```python
from build123d import *

# Parameters (mm, degrees)
F0_W     = 482.6
F0_H     = 76.2
F1_DEPTH = 6.35
F2_W     = 25.4
F2_H     = 6.35
F3_DEPTH = 6.35
F4_W     = 6.35
F4_H     = 12.7
F5_DEPTH = 6.35


with BuildPart() as f1:
    # F0 (on Right) → F1 (new body)
    with BuildSketch(Plane.YZ):
        Rectangle(F0_W, F0_H)
    extrude(amount=F1_DEPTH)

    # F2 (on face) → F3 (cut, through all)
    with BuildSketch(Plane.YZ.offset(6.35)):
        with Locations((-228.6, -34.925)):
            Rectangle(F2_W, F2_H)
        with Locations((-177.8, -34.925)):
            Rectangle(F2_W, F2_H)
        with Locations((-127, -34.925)):
            Rectangle(F2_W, F2_H)
        with Locations((-76.2, -34.925)):
            Rectangle(F2_W, F2_H)
        with Locations((-25.4, -34.925)):
            Rectangle(F2_W, F2_H)
        with Locations((25.4, -34.925)):
            Rectangle(F2_W, F2_H)
        with Locations((76.2, -34.925)):
            Rectangle(F2_W, F2_H)
        with Locations((127, -34.925)):
            Rectangle(F2_W, F2_H)
        with Locations((177.8, -34.925)):
            Rectangle(F2_W, F2_H)
        with Locations((228.6, -34.925)):
            Rectangle(F2_W, F2_H)
    extrude(amount=-F3_DEPTH, mode=Mode.SUBTRACT)

    # F4 (on face) → F5 (cut, through all)
    with BuildSketch(Plane.YZ.offset(6.35)):
        with Locations((-238.125, 31.75)):
            Rectangle(F4_W, F4_H)
        with Locations((-238.125, 6.35)):
            Rectangle(F4_W, F4_H)
        with Locations((-238.125, -19.05)):
            Rectangle(F4_W, F4_H)
        with Locations((-28.575, 31.75)):
            Rectangle(F4_W, F4_H)
        with Locations((-28.575, 6.35)):
            Rectangle(F4_W, F4_H)
        with Locations((-28.575, -19.05)):
            Rectangle(F4_W, F4_H)
        with Locations((238.125, 31.75)):
            Rectangle(F4_W, F4_H)
        with Locations((238.125, 6.35)):
            Rectangle(F4_W, F4_H)
        with Locations((238.125, -19.05)):
            Rectangle(F4_W, F4_H)
    extrude(amount=-F5_DEPTH, mode=Mode.SUBTRACT)


solid = f1.part
```
Model file for the job. Use its own axes, mm. Give positions to 0.01 mm unless a question says otherwise; leave off trailing zeros. Write each loop counter-clockwise with the first axis right and the second up, starting at its lowest first coordinate (ties: lowest second). Pieces come first, ordered by that corner, then holes. Notation, with made-up numbers: (-26.75, -29.5) -> (-20.75, -29.5) arc R11 ccw to (-20.75, -14.5) -> close; hole circle Ø10 at (-0.5, -37). An arc over 180 degrees is marked (long way). Use CSV: the item, a comma, the result in double quotes. Start each with the question number.
1) Pin check, flat tips, straight feed: P1, Ø3, axis at x = 2.5, z = -22, coming from the -Y side; P2, Ø10, axis at y = 105, z = 12, coming from the -X side; P3, Ø1.9, axis at x = 2, y = -27, coming from the -Z side; P4, Ø1.9, axis at x = 4, y = -28.5, coming from the +Z side. Stop position of each tip, or through.
2) Drill centre lines: L1, parallel to Y at x = 1, z = 3; L2, parallel to Z at x = 3, y = 13.5. Where is each one in solid material? Low to high.
3) Cut at C-C on y = 29. List the corners of the cut face in (x, z), plus the area to 3 significant figures.
4) Cut at B-B on x = 5.25. Count the separate pieces of the cut face and the enclosed holes in it, plus the area to 3 significant figures.
5) Cut at A-A on z = -17.5. List the corners of the cut face in (x, y).
Final values:
1,P1,"stops at y = -234.95"
1,P2,"stops at x = 0"
1,P3,"stops at z = -31.75"
1,P4,"stops at z = 25.4"
2,L1,"y = -234.95 to -31.75, -25.4 to 234.95"
2,L2,"z = -31.75 to 38.1"
3,outline,"(0, -31.75) -> (6.35, -31.75) -> (6.35, 38.1) -> (0, 38.1) -> close"
3,area,"444 mm2"
4,separate pieces,"1"
4,enclosed holes,"2"
4,area,"34,400 mm2"
5,outline,"(0, -234.95) -> (6.35, -234.95) -> (6.35, -31.75) -> (0, -31.75) -> close; (0, -25.4) -> (6.35, -25.4) -> (6.35, 234.95) -> (0, 234.95) -> close"
